Part print with two shaded views. Sizes in mm from the minimum x, y, z corner. Round coordinates to 2 decimals unless told otherwise and drop trailing zeros. Write each loop counter-clockwise with the first axis right and the second up, starting at its lowest first coordinate (ties: lowest second). Pieces come first, ordered by that corner, then holes. Notation, with made-up numbers: M -4,71.25 L 25,71.25 A8 cw 25,76.25 Z; hole C 50.5,60.5 d6. An arc over 180 degrees is marked long. Use one line per item in the form item = value. Start each with the question number.
Item 1: Probe L1, parallel to Y at x = 9, z = 7.25; L2, parallel to Z at x = 2.5, y = 4.4. List the from-to ranges inside material, lowest first.
Item 2: Cut at D-D, the plane x = 3. Give the cut face in (y, z), then the cut area to 3 significant figures.
Item 3: Cut at A-A, the plane z = 7.75. State how many separate pieces and enclosed holes the cut face has.
Item 4: Cut at B-B, the plane x = 6.5. Give the cut face in (y, z).
Item 5: Cut at C-C, the plane y = 3.3. Give the cut face in (x, z), then the cut area to 3 significant figures.
Item 6: Flat gauge pins, fed straight in: pin 1 Ø0.7 at (y, z) = (4, 10.5) entering from +X; pin 2 Ø1 at (x, z) = (4, 8) entering from +Y; pin 3 Ø0.7 at (x, z) = (1.5, 1.5) entering from -Y. Where does each tip first touch, or does it go through?
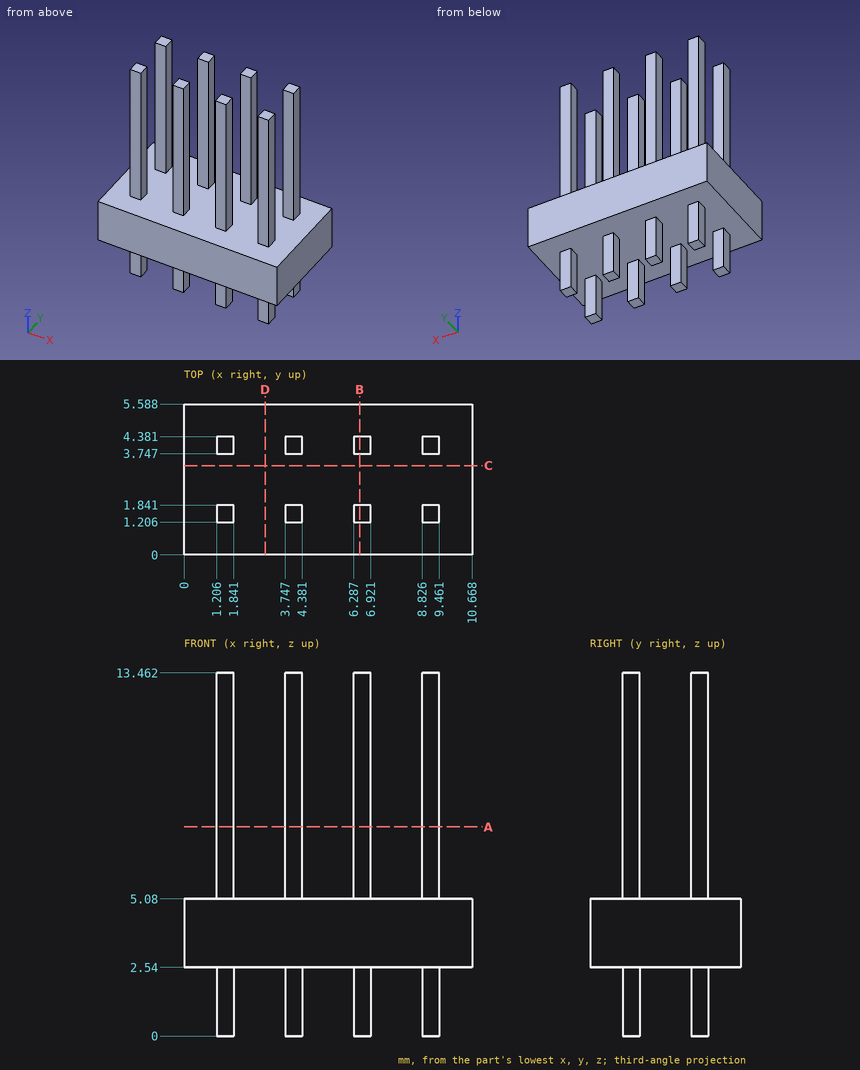
Model answer:
q1.L1 = 1.21 to 1.84, 3.75 to 4.38
q1.L2 = 2.54 to 5.08
q2.outline = M 0,2.54 L 5.59,2.54 L 5.59,5.08 L 0,5.08 Z
q2.area = 14.2 mm²
q3.separate_pieces = 8
q3.enclosed_holes = 0
q4.outline = M 0,2.54 L 1.21,2.54 L 1.21,0 L 1.84,0 L 1.84,2.54 L 3.75,2.54 L 3.75,0 L 4.38,0 L 4.38,2.54 L 5.59,2.54 L 5.59,5.08 L 4.38,5.08 L 4.38,13.46 L 3.75,13.46 L 3.75,5.08 L 1.84,5.08 L 1.84,13.46 L 1.21,13.46 L 1.21,5.08 L 0,5.08 Z
q5.outline = M 0,2.54 L 10.67,2.54 L 10.67,5.08 L 0,5.08 Z
q5.area = 27.1 mm²
q6.pin_1 = 9.46
q6.pin_2 = 4.38
q6.pin_3 = 1.21
